CAD build for the part. Positions are in the model's coordinates, mm. Face numbers are marked on the shaded views. A direction names the side the tool comes from. Give positions to 0.01 mm unless a question says otherwise; leave off trailing zeros. Order: outer loops, then holes, each group sorted by start corner. A loop starts at its lowest first (then second) coordinate and runs counter-clockwise, first axis right, second up. Notation, with made-up numbers: (42, 7.5) -> (75, 7.5) arc R24 ccw to (75, 39.5) -> close; hole circle Ø10 at (31, -13.5). An arc over 180 degrees is marked (long way). Use one line per item in the form item = value. Start each with the question number.
1) Cut at C-C, the plane x = -45. Give the cut face in (y, z).
2) Mould opens along Y. For the marked faces 1, 2 and 3 say: pulls with the +Y half, pulls with the -Y half, needs draft (parallel to the pull), parting line crosses it, or undercut.
3) Tool access for the marked faces 4 and 5: list every direction of +Z, -Z, +X, -X, +Y, -Y with a clear straight run to the whole face (end or side of a thin tool).
4) Drop flat-ended pins along their axis: P1, Ø12, axis at x = 37, y = -10, coming from the -Z side; P2, Ø23, axis at x = -51.16, y = 0, coming from the -Z side. Give the stop position or say it passes through.
5) Cut at A-A, the plane y = -17. Give the cut face in (x, z), and give its area (3 significant figures).
6) Cut at D-D, the plane y = 5.5. State how many separate pieces and enclosed holes the cut face has, and give its area (3 significant figures).
7) Cut at B-B, the plane z = -69. Give the cut face in (x, y).
8) Probe line 1 (Z direction, x = 64, y = -6); line 2 (X direction, y = 8, z = 9.5); line 3 (Y direction, x = 51.5, z = -30). List the from-to ranges inside material, lowest first.
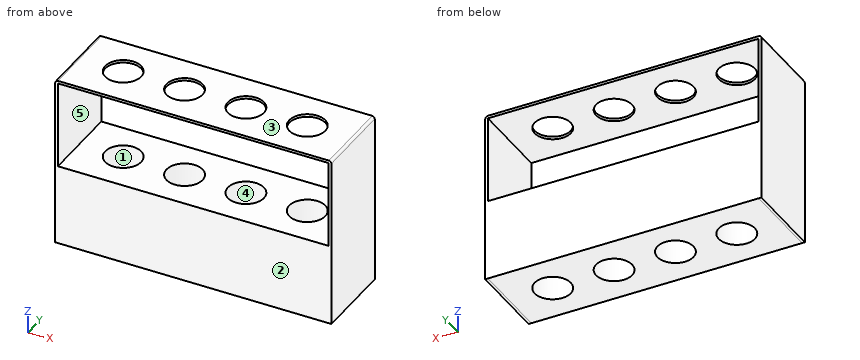
from build123d import *

# Parameters (mm, degrees)
F1_DEPTH = 22.5
F2_DEPTH = 22.5
F3_DEPTH = 22.5
F4_DEPTH = 22.5
F6_D     = 20


with BuildPart() as f1:
    # F0 (on Front) → F1 (new body)
    with BuildSketch(Plane.XZ):
        Polygon((-75.2860918641, -29.9065916457), (-75.2860918641, -74.9065916457), (74.7139081359, -75.1878393225), (74.7139081359, -29.9065916457), align=None)
    extrude(amount=F1_DEPTH)

    # F2 (add): a face of the model
    f2_faces = [f1.faces().sort_by_distance(p)[0] for p in [
        (-0.2082108855, 0, -52.4769765777),
    ]]
    extrude(f2_faces, amount=F2_DEPTH)

    # F0 (on Front) → F3 (join)
    with BuildSketch(Plane.XZ):
        with BuildLine():
            Line((-76.7860918641, -74.9065916457), (-75.2860918641, -74.9065916457))
            Line((-75.2860918641, -74.9065916457), (-75.2860918641, -29.9065916457))
            Line((-75.2860918641, -29.9065916457), (-75.2860918641, 18.5934083543))
            Line((-75.2860918641, 18.5934083543), (74.7139081359, 18.5934083543))
            Line((74.7139081359, 18.5934083543), (74.7139081359, -29.9065916457))
            Line((74.7139081359, -29.9065916457), (74.7139081359, -75.1878393225))
            Line((74.7139081359, -75.1878393225), (76.2139081359, -75.1878393225))
            Line((76.2139081359, -75.1878393225), (76.2139081359, -29.9065916457))
            Line((76.2139081359, -29.9065916457), (76.2139081359, 18.4646829894))
            Line((76.2139081359, 18.4646829894), (76.2139081359, 18.7221337192))
            ThreePointArc((76.2139081359, 18.7221337192), (75.7784667814, 19.6579669998), (74.8426335008, 20.0934083543))
            Line((74.8426335008, 20.0934083543), (74.7139081359, 20.0934083543))
            Line((74.7139081359, 20.0934083543), (74.585182771, 20.0934083543))
            Line((74.585182771, 20.0934083543), (-75.2860918641, 20.0934083543))
            ThreePointArc((-75.2860918641, 20.0934083543), (-76.3467520359, 19.6540685261), (-76.7860918641, 18.5934083543))
            Line((-76.7860918641, 18.5934083543), (-76.7860918641, -29.9065916457))
            Line((-76.7860918641, -29.9065916457), (-76.7860918641, -74.9065916457))
        make_face()
    extrude(amount=F3_DEPTH)

    # F0 (on Front) → F4 (join)
    with BuildSketch(Plane.XZ):
        with BuildLine():
            Line((-76.7860918641, -74.9065916457), (-75.2860918641, -74.9065916457))
            Line((-75.2860918641, -74.9065916457), (-75.2860918641, -29.9065916457))
            Line((-75.2860918641, -29.9065916457), (-75.2860918641, 18.5934083543))
            Line((-75.2860918641, 18.5934083543), (74.7139081359, 18.5934083543))
            Line((74.7139081359, 18.5934083543), (74.7139081359, -29.9065916457))
            Line((74.7139081359, -29.9065916457), (74.7139081359, -75.1878393225))
            Line((74.7139081359, -75.1878393225), (76.2139081359, -75.1878393225))
            Line((76.2139081359, -75.1878393225), (76.2139081359, -29.9065916457))
            Line((76.2139081359, -29.9065916457), (76.2139081359, 18.4646829894))
            Line((76.2139081359, 18.4646829894), (76.2139081359, 18.7221337192))
            ThreePointArc((76.2139081359, 18.7221337192), (75.7784667814, 19.6579669998), (74.8426335008, 20.0934083543))
            Line((74.8426335008, 20.0934083543), (74.7139081359, 20.0934083543))
            Line((74.7139081359, 20.0934083543), (74.585182771, 20.0934083543))
            Line((74.585182771, 20.0934083543), (-75.2860918641, 20.0934083543))
            ThreePointArc((-75.2860918641, 20.0934083543), (-76.3467520359, 19.6540685261), (-76.7860918641, 18.5934083543))
            Line((-76.7860918641, 18.5934083543), (-76.7860918641, -29.9065916457))
            Line((-76.7860918641, -29.9065916457), (-76.7860918641, -74.9065916457))
        make_face()
    extrude(amount=-F4_DEPTH)

    # F6 (through all)
    with Locations(Plane.XY.offset(20.0934083543)):
        with Locations((-51.1573664992, 0), (-17.1573664992, 0), (16.8426335008, 0), (50.8426335008, 0)):
            Hole(F6_D / 2)


solid = f1.part
Result:
q1.outline = (-22.5, -74.96) -> (-7.88, -74.96) -> (-7.88, -29.91) -> (-22.5, -29.91) -> close; (-22.5, 18.59) -> (-7.88, 18.59) -> (-7.88, 20.09) -> (-22.5, 20.09) -> close; (7.88, -74.96) -> (22.5, -74.96) -> (22.5, -29.91) -> (7.88, -29.91) -> close; (7.88, 18.59) -> (22.5, 18.59) -> (22.5, 20.09) -> (7.88, 20.09) -> close
q2.face_1 = undercut
q2.face_2 = pulls with the -Y half
q2.face_3 = needs draft
q3.face_4 = +Z, -Z
q3.face_5 = +Y, -Y
q4.P1 = -75.13
q4.P2 = -74.97
q5.outline = (-76.79, -74.91) -> (-75.29, -74.91) -> (74.71, -75.19) -> (76.21, -75.19) -> (76.21, 18.72) arc R1.51 ccw to (74.84, 20.09) -> (-75.29, 20.09) arc R1.5 ccw to (-76.79, 18.59) -> close; hole (-75.29, -29.91) -> (74.71, -29.91) -> (74.71, 18.59) -> (-75.29, 18.59) -> close
q5.area = 7,280 mm²
q6.separate_pieces = 8
q6.enclosed_holes = 0
q6.area = 4,160 mm²
q7.outline = (-76.79, -22.5) -> (76.21, -22.5) -> (76.21, 22.5) -> (-76.79, 22.5) -> close; hole circle Ø20 at (-51.16, 0); hole circle Ø20 at (-17.16, 0); hole circle Ø20 at (16.84, 0); hole circle Ø20 at (50.84, 0)
q8.line_1 = -75.17 to -29.91, 18.59 to 20.09
q8.line_2 = -76.79 to -75.29, 74.71 to 76.21
q8.line_3 = -22.5 to -9.98, 9.98 to 22.5
